Could you check a few things on this model? Use its own coordinates, in mm. A direction names the side the tool comes from. Give positions to 0.01 mm unless a question says otherwise; leave off trailing zeros. Loops run counter-clockwise (first coordinate to the right, second up) from the corner with the lowest first, then second, coordinate; pieces in that order, holes last. Notation, with made-up numbers: M -14,-3 L -9,-3 A23 cw -9,5 Z; hole C 36.25,3 d8. An arc over 180 degrees is marked long. Answer in a Markdown table with one row per item. Add a question column.
```python
from build123d import *

# Parameters (mm, degrees)
SKETCH1_W           = 20
SKETCH1_H           = 15
BOSS_EXTRUDE3_DEPTH = 3
SKETCH4_W           = 13
SKETCH4_H           = 1.5
CUT_EXTRUDE1_DEPTH  = 18
SKETCH5_W           = 7.5
SKETCH5_H           = 10
CUT_EXTRUDE2_DEPTH  = 18
SKETCH5_3_W         = 1
SKETCH5_3_H         = 15
CUT_EXTRUDE3_DEPTH  = 18


with BuildPart() as part:
    # Sketch1 → Boss-Extrude3 (new body)
    with BuildSketch(Plane(origin=(0, 0, 0), x_dir=(1, 0, 0), z_dir=(0, 1, 0))):
        Rectangle(SKETCH1_W, SKETCH1_H)
    extrude(amount=BOSS_EXTRUDE3_DEPTH)

    # Sketch4 → Cut-Extrude1 (cut)
    with BuildSketch(Plane.ZY.offset(10)):
        with Locations((0, 1.5)):
            Rectangle(SKETCH4_W, SKETCH4_H)
    extrude(amount=-CUT_EXTRUDE1_DEPTH, mode=Mode.SUBTRACT)

    # Sketch5 → Cut-Extrude2 (cut)
    with BuildSketch(Plane(origin=(0, 3, 0), x_dir=(1, 0, 0), z_dir=(0, 1, 0))):
        with Locations((-4.75, 0)):
            Rectangle(SKETCH5_W, SKETCH5_H)
        with Locations((2.75, 0)):
            Rectangle(SKETCH5_W, SKETCH5_H)
    extrude(amount=-CUT_EXTRUDE2_DEPTH, mode=Mode.SUBTRACT)

    # Sketch5_3 → Cut-Extrude3 (cut)
    with BuildSketch(Plane(origin=(0, 3, 0), x_dir=(1, 0, 0), z_dir=(0, 1, 0))):
        with Locations((9.5, 0)):
            Rectangle(SKETCH5_3_W, SKETCH5_3_H)
    extrude(amount=-CUT_EXTRUDE3_DEPTH, mode=Mode.SUBTRACT)


solid = part.part
```
Item 1: Suppose I cut it at B-B (y = 0.25). List the corners of the cut face in (x, z) for me, then the cut area to 3 significant figures.
Item 2: For faces 1 (the face through (-1, 2.25, -6)), 2 (the face through (-1, 1, 7.5)), which set-ups out of +Z, -Z, +X, -X, +Y, -Y let a thin tool reach every point of the face, with its end or its side?
Item 3: Suppose I cut it at D-D (y = 1.3). List the corners of the cut face in (x, z) for me.
Item 4: If we mould it in two halves opening along Y, with no side actions, what happens to faces 3 (the face through (-1, 0, -7)), 4 (the face through (8, 2, 0)), 5 (the face through (-1, 1, -7.5))? For each: +Y half, -Y half, draft (parallel to the pull), parting line (faces both ways), or undercut.
Item 5: Suppose I cut it at C-C (z = -2.5). List the corners of the cut face in (x, y) for me.
Item 6: I need wall thicknesses on L1, parallel to X at y = 0.35, z = -2.25; L2, parallel to Z at x = -7.75, y = 2.05; L3, parallel to Y at x = -8.75, z = -2. Which ranges of each line are inside material? Lowest first, please.
Item 7: Suppose I cut it at A-A (x = -4.75). List the corners of the cut face in (y, z) for me, then the cut area to 3 significant figures.
Values found:
| question | item | result |
|---|---|---|
| 1 | outline | M -10,-7.5 L 9,-7.5 L 9,7.5 L -10,7.5 Z; hole M -8.5,-5 L 6.5,-5 L 6.5,5 L -8.5,5 Z |
| 1 | area | 135 mm² |
| 2 | face 1 | -X |
| 2 | face 2 | +Z, +X, -X, +Y, -Y |
| 3 | outline | M -10,-7.5 L 9,-7.5 L 9,7.5 L -10,7.5 L -10,6.5 L 8,6.5 L 8,-6.5 L -10,-6.5 Z |
| 4 | face 3 | -Y half |
| 4 | face 4 | undercut |
| 4 | face 5 | draft |
| 5 | outline | M -10,0 L -8.5,0 L -8.5,0.75 L -10,0.75 Z; M -10,2.25 L -8.5,2.25 L -8.5,3 L -10,3 Z; M 6.5,0 L 9,0 L 9,3 L 6.5,3 L 6.5,2.25 L 8,2.25 L 8,0.75 L 6.5,0.75 Z |
| 6 | L1 | -10 to -8.5, 6.5 to 9 |
| 6 | L2 | -7.5 to -6.5, 6.5 to 7.5 |
| 6 | L3 | 0 to 0.75, 2.25 to 3 |
| 7 | outline | M 0,-7.5 L 3,-7.5 L 3,-5 L 2.25,-5 L 2.25,-6.5 L 0.75,-6.5 L 0.75,-5 L 0,-5 Z; M 0,5 L 0.75,5 L 0.75,6.5 L 2.25,6.5 L 2.25,5 L 3,5 L 3,7.5 L 0,7.5 Z |
| 7 | area | 10.5 mm² |
